```python
from build123d import *

# Parameters (mm, degrees)
SKETCH121_R             = 6
PAD085_DEPTH            = 3
SKETCH122_W             = 26
SKETCH122_H             = 3
PAD086_DEPTH            = 30
SKETCH123_R             = 2
POCKET048_DEPTH         = 30.001
SKETCH124_R             = 1
POCKET049_DEPTH         = 136.248276
POLARPATTERN018_COUNT   = 4
BODY050_PLACEMENT_ANGLE = 180


with BuildPart() as part:
    # Sketch121 → Pad085 (new body)
    with BuildSketch(Plane.XZ):
        with BuildLine():
            Line((-13, 17), (13, 17))
            Line((13, 17), (13, 0))
            ThreePointArc((-13, 0), (0, -13), (13, 0))
            Line((-13, 17), (-13, 0))
        make_face()
        Circle(SKETCH121_R, mode=Mode.SUBTRACT)
    extrude(amount=PAD085_DEPTH)

    # Sketch122 (on Face7 of Pad085) → Pad086 (join)
    with BuildSketch(Plane.XZ.offset(3)):
        with Locations((0, 15.5)):
            Rectangle(SKETCH122_W, SKETCH122_H)
    extrude(amount=PAD086_DEPTH)

    # Sketch123 (on Face5 of Pad086) → Pocket048 (cut, through all)
    with BuildSketch(Plane(origin=(0, 0, 17), x_dir=(-1, 0, 0), z_dir=(0, 0, 1))):
        with Locations((-9, 7)):
            Circle(SKETCH123_R)
        with Locations((9, 7)):
            Circle(SKETCH123_R)
        with Locations((-9, 29)):
            Circle(SKETCH123_R)
        with Locations((9, 29)):
            Circle(SKETCH123_R)
    extrude(amount=-POCKET048_DEPTH, mode=Mode.SUBTRACT)

    # Sketch124 (on Face4 of Pocket048) → Pocket049 (cut, through all)
    with BuildSketch(Plane(origin=(0, 0, 0), x_dir=(1, 0, 0), z_dir=(0, 1, 0))):
        with Locations((0, 9.5)):
            Circle(SKETCH124_R)
    pocket049 = extrude(amount=-POCKET049_DEPTH, mode=Mode.SUBTRACT)

    # PolarPattern018: Pocket049 ×4 about axis
    polarpattern018_axis = Axis((0, 0, 0), (0, 1, 0))
    for i in range(1, POLARPATTERN018_COUNT):
        add(pocket049.rotate(polarpattern018_axis, i * 360 / POLARPATTERN018_COUNT), mode=Mode.SUBTRACT)


with BuildPart() as part_1:
    # Body050 placement: moved
    add(part.part.moved(Location((-48.540115, 19.040115, 18))).rotate(Axis((-48.540115, 19.040115, 18), (0, 1, 0)), BODY050_PLACEMENT_ANGLE))


solid = part_1.part
```
Design review of the part built by this model. Coordinates are the model's own, in mm. Coordinates: 2 decimals unless noted, no trailing zeros. Order: outer loops, then holes, each group sorted by start corner. A loop starts at its lowest first (then second) coordinate and runs counter-clockwise, first axis right, second up.
1) Take a section at C-C, the plane y = -4.5. Give the boundary of the cut face in (x, z).
2) Mouldability with a two-part tool opening along Z and no side actions: class faces 1 (the flat face through (-48, 1, 4)), 2 (the cylindrical face through (-47.54, 17.56, 27.54)), 3 (the flat face through (-49, 16.04, 11)), 4 (the cylindrical face through (-39.93, 17.56, 18.46)) as +Z half, -Z half, draft (parallel to the pull), parting line (faces both ways), or undercut.
3) Take a section at B-B, the plane z = 13. Give the boundary of the cut face in (x, y).
4) Take a section at A-A, the plane z = 8.5. Give the boundary of the cut face in (x, y).
5) Clearance check with flat-ended pins moving along their axes: pin 1 (3 mm diameter, centred on x = -39.54, y = 12.04, fed in from +Z); pin 2 (12 mm diameter, centred on x = -58.5, z = 27.5, fed in from -Y); pin 3 (5 mm diameter, centred on x = -57.54, y = -9.96, fed in from +Z). State where each tip first meets the part, or that it passes through.
6) Wall thickness on line 1 along X through (y, z) = (17.25, 18); line 2 along Y through (x, z) = (-51, 4.5); line 3 along Z through (x, y) = (-37.5, 15): over which ranges is each line inside the solid? List them lowest first.
Returned:
1. outline: (-61.54, 1) - (-35.54, 1) - (-35.54, 4) - (-61.54, 4) - close
2. face 1: +Z half
2. face 2: undercut
2. face 3: draft
2. face 4: undercut
3. outline: (-61.54, 16.04) - (-51.86, 16.04) - (-51.86, 19.04) - (-61.54, 19.04) - close; (-45.22, 16.04) - (-35.54, 16.04) - (-35.54, 19.04) - (-45.22, 19.04) - close
4. outline: (-61.54, 16.04) - (-49.54, 16.04) - (-49.54, 19.04) - (-61.54, 19.04) - close; (-47.54, 16.04) - (-35.54, 16.04) - (-35.54, 19.04) - (-47.54, 19.04) - close
5. pin 1: passes through
5. pin 2: stops at y = 16.04
5. pin 3: stops at z = 4
6. line 1: x = -61.54 to -59.04, -57.04 to -54.54, -42.54 to -40.04, -38.04 to -35.54
6. line 2: y = 16.04 to 19.04
6. line 3: z = 1 to 4
